```python
from build123d import *

# Parameters (mm, degrees)
SKETCH1_W                = 50
SKETCH1_H                = 100
BOSS_EXTRUDE4_DEPTH      = 8.5
SKETCH2_W                = 50
SKETCH2_H                = 100
BOSS_EXTRUDE5_DEPTH      = 5
BOSS_EXTRUDE6_START      = 5
SKETCH3_W                = 50
SKETCH3_H                = 100
BOSS_EXTRUDE6_DEPTH      = 5
FILLET3_R                = 10
M5_CLEARANCE_HOLE1_D     = 5.3
M5_CLEARANCE_HOLE1_DEPTH = 15
M5_CLEARANCE_HOLE1_TIP   = 1.59228064
FILLET2_R                = 5


with BuildPart() as part:
    # Sketch1 → Boss-Extrude4 (new, symmetric)
    with BuildSketch(Plane.XY):
        with BuildLine():
            Line((0, -25), (0, 25))
            Line((0, 25), (15, 25))
            Line((15, 25), (15, 40))
            Line((15, 40), (0, 40))
            Line((0, 40), (0, 90))
            Line((0, 90), (15, 90))
            Line((15, 90), (15, 105))
            Line((15, 105), (110, 105))
            ThreePointArc((110, 105), (120.606601718, 100.606601718), (125, 90))
            Line((125, 90), (125, -90))
            ThreePointArc((125, -90), (120.606601718, -100.606601718), (110, -105))
            Line((110, -105), (15, -105))
            Line((15, -105), (15, -90))
            Line((15, -90), (0, -90))
            Line((0, -90), (0, -40))
            Line((0, -40), (15, -40))
            Line((15, -40), (15, -25))
            Line((15, -25), (0, -25))
        make_face()
        with Locations((62.5, 0)):
            Rectangle(SKETCH1_W, SKETCH1_H, mode=Mode.SUBTRACT)
    extrude(amount=BOSS_EXTRUDE4_DEPTH, both=True)

    # Sketch2 → Boss-Extrude5 (add)
    with BuildSketch(Plane(origin=(0, 0, -8.5), x_dir=(-1, 0, 0), z_dir=(0, 0, -1))):
        with BuildLine():
            Line((-110, 105), (-15, 105))
            Line((-15, 105), (-15, 90))
            Line((-15, 90), (-15, 40))
            Line((-15, 40), (-15, 25))
            Line((-15, 25), (-15, -25))
            Line((-15, -25), (-15, -40))
            Line((-15, -40), (-15, -90))
            Line((-15, -90), (-15, -105))
            Line((-15, -105), (-110, -105))
            ThreePointArc((-110, -105), (-120.606601718, -100.606601718), (-125, -90))
            Line((-125, -90), (-125, 90))
            ThreePointArc((-125, 90), (-120.606601718, 100.606601718), (-110, 105))
        make_face()
        with Locations((-62.5, 0)):
            Rectangle(SKETCH2_W, SKETCH2_H, mode=Mode.SUBTRACT)
    extrude(amount=BOSS_EXTRUDE5_DEPTH)

    # Sketch3 → Boss-Extrude6 (add)
    with BuildSketch(Plane.XY.offset(8.5).offset(BOSS_EXTRUDE6_START)):
        with BuildLine():
            Line((15, -90), (15, -105))
            Line((15, -105), (110, -105))
            ThreePointArc((110, -105), (120.606601718, -100.606601718), (125, -90))
            Line((125, -90), (125, 90))
            ThreePointArc((125, 90), (120.606601718, 100.606601718), (110, 105))
            Line((110, 105), (15, 105))
            Line((15, 105), (15, 90))
            Line((15, 90), (15, 40))
            Line((15, 40), (15, 25))
            Line((15, 25), (15, -25))
            Line((15, -25), (15, -40))
            Line((15, -40), (15, -90))
        make_face()
        with Locations((62.5, 0)):
            Rectangle(SKETCH3_W, SKETCH3_H, mode=Mode.SUBTRACT)
    extrude(amount=-BOSS_EXTRUDE6_DEPTH)

    # Fillet3
    fillet3_edges = [part.edges().sort_by_distance(p)[0] for p in [
        (37.5, 50, 0),
        (37.5, -50, 0),
        (87.5, -50, 0),
        (87.5, 50, 0),
    ]]
    fillet(fillet3_edges, radius=FILLET3_R)

    # M5 Clearance Hole1
    with Locations(Plane(origin=(62.5, 60, -13.5), x_dir=(-1, 0, 0), z_dir=(0, 0, -1))):
        with Locations((0, 0), (0, -120)):
            Hole(M5_CLEARANCE_HOLE1_D / 2, depth=M5_CLEARANCE_HOLE1_DEPTH)
            with Locations((0, 0, -(M5_CLEARANCE_HOLE1_DEPTH + M5_CLEARANCE_HOLE1_TIP / 2))):  # 118° drill point
                Cone(0, M5_CLEARANCE_HOLE1_D / 2, M5_CLEARANCE_HOLE1_TIP, mode=Mode.SUBTRACT)

    # Fillet2
    fillet2_edges = [part.edges().sort_by_distance(p)[0] for p in [
        (62.5, -105, 13.5),
        (120.606601718, -100.606601718, 13.5),
        (125, 0, 13.5),
        (120.606601718, 100.606601718, 13.5),
        (62.5, 105, 13.5),
        (120.606601718, 100.606601718, -13.5),
        (125, 0, -13.5),
        (120.606601718, -100.606601718, -13.5),
        (62.5, -105, -13.5),
        (62.5, 105, -13.5),
    ]]
    fillet(fillet2_edges, radius=FILLET2_R)


solid = part.part
```
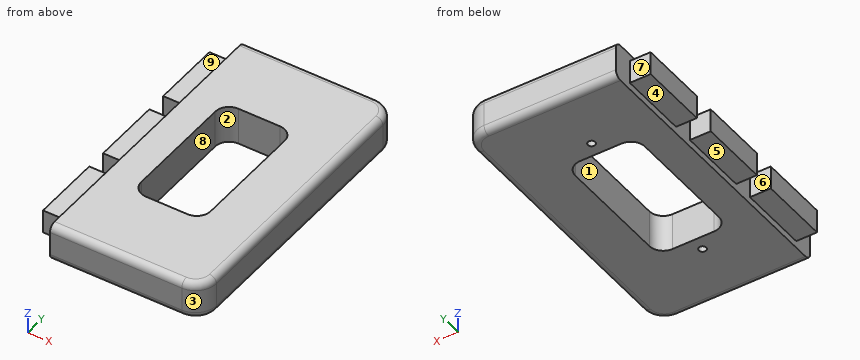
Design review of the part built by this model. Coordinates are the model's own, in mm. Face numbers are marked on the shaded views. A direction names the side the tool comes from. Coordinates: 2 decimals unless noted, no trailing zeros. Order: outer loops, then holes, each group sorted by start corner. A loop starts at its lowest first (then second) coordinate and runs counter-clockwise, first axis right, second up. Notation, with made-up numbers: (-12.75, 50.25) - (34.25, 50.25) arc R11 cw to (34.25, 67.25) - close; hole circle Ø9 at (70, 13.5). An arc over 180 degrees is marked (long way). One line per question, with ' | ' between items.
Q1. The part is to be moulded in two halves that separate along X. For the marked faces 1, 2, 3 and 4, say which applies: +X half, -X half, draft (parallel to the pull), parting line (faces both ways), or undercut.
Answer key:
face 1: undercut | face 2: undercut | face 3: +X half | face 4: draft
Q2. Consider section A-A, the plane y = 2. Give the boundary of the cut face in (x, z), then the cut area to 3 significant figures.
Answer key:
outline: (0, -8.5) - (15, -8.5) - (15, -13.5) - (37.5, -13.5) - (37.5, 13.5) - (15, 13.5) - (15, 8.5) - (0, 8.5) - close; (87.5, -13.5) - (120, -13.5) arc R5 ccw to (125, -8.5) - (125, 8.5) arc R5 ccw to (120, 13.5) - (87.5, 13.5) - close | area: 1,860 mm2
Q3. Consider section C-C, the plane z = -5.5. Give the boundary of the cut face in (x, y).
Answer key:
outline: (0, -90) - (15, -90) - (15, -105) - (110, -105) arc R15 ccw to (125, -90) - (125, 90) arc R15 ccw to (110, 105) - (15, 105) - (15, 90) - (0, 90) - (0, 40) - (15, 40) - (15, 25) - (0, 25) - (0, -25) - (15, -25) - (15, -40) - (0, -40) - close; hole (37.5, -40) arc R10 ccw to (47.5, -50) - (77.5, -50) arc R10 ccw to (87.5, -40) - (87.5, 40) arc R10 ccw to (77.5, 50) - (47.5, 50) arc R10 ccw to (37.5, 40) - close; hole circle Ø5.3 at (62.5, -60); hole circle Ø5.3 at (62.5, 60)
Q4. For the marked faces 5, 6, 7, 8 and 9, list the 3-axis set-ups (+Z, -Z, +X, -X, +Y, -Y) from which the entire face can be reached by the end or side of a thin tool; tool diameter is ignored.
Answer key:
face 5: -Z, -X, +Y, -Y | face 6: +Z, -Z, -X | face 7: +Z, -Z, -X, +Y | face 8: +Z, -Z | face 9: +Z, -X, +Y, -Y
Q5. To check wall thickness, follow line 1 along Y through (x, z) = (62.5, -8.25); line 2 along Y through (x, z) = (9, 2.5); line 3 along X through (y, z) = (60, -7.25). State the ranges of each line that lie inside material, in increasing order.
Answer key:
line 1: y = -105 to -62.65, -57.35 to -50, 50 to 57.35, 62.65 to 105 | line 2: y = -90 to -40, -25 to 25, 40 to 90 | line 3: x = 0 to 59.85, 65.15 to 125
Q6. Consider section B-B, the plane x = 8. Give the boundary of the cut face in (y, z).
Answer key:
outline: (-90, -8.5) - (-40, -8.5) - (-40, 8.5) - (-90, 8.5) - close; (-25, -8.5) - (25, -8.5) - (25, 8.5) - (-25, 8.5) - close; (40, -8.5) - (90, -8.5) - (90, 8.5) - (40, 8.5) - close
Q7. Consider section D-D, the plane y = -87. Give the boundary of the cut face in (x, z), then the cut area to 3 significant figures.
Answer key:
outline: (0, -8.5) - (15, -8.5) - (15, -13.5) - (120, -13.5) arc R5 ccw to (125, -8.5) - (125, 8.5) arc R5 ccw to (120, 13.5) - (15, 13.5) - (15, 8.5) - (0, 8.5) - close | area: 3,210 mm2
Q8. Clearance check with flat-ended pins moving along their axes: pin 1 Ø7.5 at (x, z) = (8, -1) entering from -Y; pin 2 Ø5 at (x, y) = (62.5, -60) entering from -Z; pin 3 Ø4.5 at (x, z) = (4.5, -2.5) entering from +Y. State where each tip first meets the part, or that it passes through.
Answer key:
pin 1: stops at y = -90 | pin 2: stops at z = 1.59 | pin 3: stops at y = 90
